```python
from build123d import *

# Parameters (mm, degrees)
EXTRUDE_1_DEPTH          = 20
CUT_EXTRUDE_1_DEPTH      = 83.680748207
CUT_EXTRUDE_1_DEPTH_BACK = 83.680748207
SKETCH_2_R               = 1.1
FILLET_1_R               = 1


with BuildPart() as part:
    # 草图1 → 凸台-拉伸1 (new body)
    with BuildSketch(Plane(origin=(0, 0, 0), x_dir=(1, 0, 0), z_dir=(0, 1, 0))):
        with BuildLine():
            Line((67.351218567, -14.287180049), (67.351218567, -15.287180049))
            Line((67.351218567, -15.287180049), (70.414699146, -15.287180049))
            ThreePointArc((70.414699146, -15.287180049), (73.768801112, -17.787180049), (77.122903079, -15.287180049))
            Line((77.122903079, -15.287180049), (80.186383657, -15.287180049))
            Line((80.186383657, -15.287180049), (80.186383657, -14.287180049))
            Line((80.186383657, -14.287180049), (75.823885018, -14.287180049))
            ThreePointArc((75.823885018, -14.287180049), (73.771343065, -16.339722002), (71.718801112, -14.287180049))
            Line((71.718801112, -14.287180049), (67.351218567, -14.287180049))
        make_face()
    extrude(amount=EXTRUDE_1_DEPTH)

    # 草图2 → 切除-拉伸1 (cut, two sides: drawn at the far end of the back side and taken through both)
    with BuildSketch(Plane.XY.offset(15.287180049).offset(-CUT_EXTRUDE_1_DEPTH_BACK)):
        with Locations((68.921019173, 18.327295742)):
            Circle(SKETCH_2_R)
        with Locations((68.921019173, 1.629689565)):
            Circle(SKETCH_2_R)
        with Locations((78.60655426, 18.327295742)):
            Circle(SKETCH_2_R)
        with Locations((78.60655426, 1.629689565)):
            Circle(SKETCH_2_R)
    extrude(amount=CUT_EXTRUDE_1_DEPTH + CUT_EXTRUDE_1_DEPTH_BACK, mode=Mode.SUBTRACT)

    # 圆角1
    fillet_1_edges = [part.edges().sort_by_distance(p)[0] for p in [
        (80.186383657, 20, 14.787180049),
        (67.351218567, 20, 14.787180049),
        (67.351218567, 0, 14.787180049),
        (80.186383657, 0, 14.787180049),
    ]]
    fillet(fillet_1_edges, radius=FILLET_1_R)


solid = part.part
```
The model under review builds one solid part; all positions refer to its coordinate system, in mm. A direction names the side the tool comes from. Round coordinates to 2 decimals unless told otherwise and drop trailing zeros. Loops run counter-clockwise (first coordinate to the right, second up) from the corner with the lowest first, then second, coordinate; pieces in that order, holes last.
Item 1: For faces 4 (the face through (67.351, 10, 15)), 5 (the face through (69, 10, 15.287)), list the 3-axis set-ups (+Z, -Z, +X, -X, +Y, -Y) from which the entire face can be reached by the end or side of a thin tool; tool diameter is ignored.
Determined:
face 4: +Z, -Z, -X, +Y, -Y
face 5: +Z, -X, +Y, -Y
Item 2: Take a section at B-B (y = 3.5). Write out the cut boundary in (x, z), then the cut area to 3 significant figures.
Determined:
outline: (67.35, 14.29) - (71.72, 14.29) arc R2.05 cw to (75.82, 14.29) - (80.19, 14.29) - (80.19, 15.29) - (77.12, 15.29) arc R3.5 ccw to (70.41, 15.29) - (67.35, 15.29) - close
area: 18.6 mm2
Item 3: Take a section at A-A (z = 14.9). Write out the cut boundary in (x, y).
Determined:
outline: (67.35, 1) arc R1 ccw to (68.35, 0) - (71.81, 0) - (71.81, 20) - (68.35, 20) arc R1 ccw to (67.35, 19) - close; (75.73, 0) - (79.19, 0) arc R1 ccw to (80.19, 1) - (80.19, 19) arc R1 ccw to (79.19, 20) - (75.73, 20) - close; hole circle Ø2.2 at (68.92, 1.63); hole circle Ø2.2 at (68.92, 18.33); hole circle Ø2.2 at (78.61, 1.63); hole circle Ø2.2 at (78.61, 18.33)
Item 4: Take a section at D-D (z = 15.8). Write out the cut boundary in (x, y).
Determined:
outline: (70.61, 0) - (72.38, 0) - (72.38, 20) - (70.61, 20) - close; (75.16, 0) - (76.92, 0) - (76.92, 20) - (75.16, 20) - close
Item 5: For line 1 (Z direction, x = 79.5, y = 4.25); line 2 (X direction, y = 1, z = 14.6); line 3 (X direction, y = 5.75, z = 15.4), list the stretches that pass through material, from the lowest coordinate up.
Determined:
line 1: z = 14.29 to 15.29
line 2: x = 67.35 to 68.02, 69.82 to 71.74, 75.8 to 77.7, 79.51 to 80.19
line 3: x = 70.45 to 72.05, 75.5 to 77.09
Item 6: Mouldability with a two-part tool opening along Y and no side actions: class faces 1 (the face through (79.9, 19.7, 14.8)), 2 (the face through (79, 10, 15.287)), 3 (the face through (67.822, 1.678, 14.78)) as released by +Y, released by -Y, zero draft, split by the parting line, or undercut.
Determined:
face 1: released by +Y
face 2: zero draft
face 3: undercut
Item 7: Take a section at C-C (x = 78.5). Write out the cut boundary in (y, z).
Determined:
outline: (0, 14.29) - (0.53, 14.29) - (0.53, 15.29) - (0, 15.29) - close; (2.72, 14.29) - (17.23, 14.29) - (17.23, 15.29) - (2.72, 15.29) - close; (19.42, 14.29) - (20, 14.29) - (20, 15.29) - (19.42, 15.29) - close
Item 8: Clearance check with flat-ended pins moving along their axes: pin 1 Ø1.8 at (x, y) = (68.92, 1.63) entering from -Z; pin 2 Ø1 at (x, y) = (71, 13) entering from +Z; pin 3 Ø2.5 at (x, y) = (69.5, 14.5) entering from +Z; pin 4 Ø0.9 at (x, y) = (79, 7) entering from +Z. State where each tip first meets the part, or that it passes through.
Determined:
pin 1: passes through
pin 2: stops at z = 16.95
pin 3: stops at z = 16.06
pin 4: stops at z = 15.29
